Model file for the job. Use its own axes, mm. A direction names the side the tool comes from. Coordinates: 2 decimals unless noted, no trailing zeros. Order: outer loops, then holes, each group sorted by start corner. A loop starts at its lowest first (then second) coordinate and runs counter-clockwise, first axis right, second up. Notation, with made-up numbers: (4, 48.5) -> (10, 48.5) arc R25 ccw to (10, 83.5) -> close; hole circle Ø7 at (-17, 8.25). An arc over 180 degrees is marked (long way). Return JSON: item names as keys, results as strings. Group by question number.
1) Probe line 1 (Y direction, x = 31, z = 95); line 2 (Z direction, x = 273, y = 10.5) (3 decimals); line 3 (Y direction, x = 35.5, z = 82). List the from-to ranges inside material, lowest first.
2) Which spindle directions (+Z, -Z, +X, -X, +Y, -Y) get a long thin tool onto all of the face, cutting with end or side? Do faces 1 (the flat face through (302, -1, 0)), 2 (the flat face through (-10, 10, 0)), 3 (the flat face through (455, -10, 0)), 4 (the flat face through (454, 10, 127)). Say none if no direction does.
3) Flat gauge pins, fed straight in: pin 1 (1.5 mm diameter, centred on x = 292, z = 116, fed in from -Y); pin 2 (2 mm diameter, centred on y = -8.5, z = 73, fed in from +X); pin 3 (4 mm diameter, centred on x = -4, y = -5.5, fed in from +Z) (3 decimals); pin 4 (4 mm diameter, centred on x = 79.5, z = 90.5, fed in from +Y). Where does each tip first touch, or does it go through?
4) Cut at B-B (x = 120.5). Write the cut outline in (y, z) (3 decimals).
5) Pull direction X, two halves, no side cores. Call faces 5 (the flat face through (111, -1, 127)), 6 (the flat face through (219, 0, 130.175)): +X half, -X half, draft (parallel to the pull), parting line (faces both ways), or undercut.
6) Cut at A-A (z = 67). State how many separate pieces and enclosed holes the cut face has, and give its area (3 significant figures).
from build123d import *

# Parameters (mm, degrees)
SKETCH1_R           = 12.7
BOSS_EXTRUDE1_DEPTH = 127
LPATTERN1_COUNT     = 15
LPATTERN1_PITCH     = 31.75
SKETCH2_W           = 469.9
SKETCH2_H           = 25.4
BOSS_EXTRUDE2_DEPTH = 3.175
SKETCH3_R           = 8.255
CUT_EXTRUDE1_DEPTH  = 477.41930324


with BuildPart() as part:
    # Sketch1 → Boss-Extrude1 (new body)
    with BuildSketch(Plane.XY):
        Circle(SKETCH1_R)
    extrude(amount=BOSS_EXTRUDE1_DEPTH)


with BuildPart() as lpattern1_1:
    # LPattern1: pattern copy
    add(part.part.moved(Location(Vector(1, 0, 0) * (1 * LPATTERN1_PITCH))))


with BuildPart() as lpattern1_2:
    # LPattern1: pattern copy
    add(part.part.moved(Location(Vector(1, 0, 0) * (2 * LPATTERN1_PITCH))))


with BuildPart() as lpattern1_3:
    # LPattern1: pattern copy
    add(part.part.moved(Location(Vector(1, 0, 0) * (3 * LPATTERN1_PITCH))))


with BuildPart() as lpattern1_4:
    # LPattern1: pattern copy
    add(part.part.moved(Location(Vector(1, 0, 0) * (4 * LPATTERN1_PITCH))))


with BuildPart() as lpattern1_5:
    # LPattern1: pattern copy
    add(part.part.moved(Location(Vector(1, 0, 0) * (5 * LPATTERN1_PITCH))))


with BuildPart() as lpattern1_6:
    # LPattern1: pattern copy
    add(part.part.moved(Location(Vector(1, 0, 0) * (6 * LPATTERN1_PITCH))))


with BuildPart() as lpattern1_7:
    # LPattern1: pattern copy
    add(part.part.moved(Location(Vector(1, 0, 0) * (7 * LPATTERN1_PITCH))))


with BuildPart() as lpattern1_8:
    # LPattern1: pattern copy
    add(part.part.moved(Location(Vector(1, 0, 0) * (8 * LPATTERN1_PITCH))))


with BuildPart() as lpattern1_9:
    # LPattern1: pattern copy
    add(part.part.moved(Location(Vector(1, 0, 0) * (9 * LPATTERN1_PITCH))))


with BuildPart() as lpattern1_10:
    # LPattern1: pattern copy
    add(part.part.moved(Location(Vector(1, 0, 0) * (10 * LPATTERN1_PITCH))))


with BuildPart() as lpattern1_11:
    # LPattern1: pattern copy
    add(part.part.moved(Location(Vector(1, 0, 0) * (11 * LPATTERN1_PITCH))))


with BuildPart() as lpattern1_12:
    # LPattern1: pattern copy
    add(part.part.moved(Location(Vector(1, 0, 0) * (12 * LPATTERN1_PITCH))))


with BuildPart() as lpattern1_13:
    # LPattern1: pattern copy
    add(part.part.moved(Location(Vector(1, 0, 0) * (13 * LPATTERN1_PITCH))))


with BuildPart() as lpattern1_14:
    # LPattern1: pattern copy
    add(part.part.moved(Location(Vector(1, 0, 0) * (14 * LPATTERN1_PITCH))))


with BuildPart() as part_1:
    add(part.part)

    add(lpattern1_1.part)  # Boss-Extrude2 merges LPattern1_1

    add(lpattern1_2.part)  # Boss-Extrude2 merges LPattern1_2

    add(lpattern1_3.part)  # Boss-Extrude2 merges LPattern1_3

    add(lpattern1_4.part)  # Boss-Extrude2 merges LPattern1_4

    add(lpattern1_5.part)  # Boss-Extrude2 merges LPattern1_5

    add(lpattern1_6.part)  # Boss-Extrude2 merges LPattern1_6

    add(lpattern1_7.part)  # Boss-Extrude2 merges LPattern1_7

    add(lpattern1_8.part)  # Boss-Extrude2 merges LPattern1_8

    add(lpattern1_9.part)  # Boss-Extrude2 merges LPattern1_9

    add(lpattern1_10.part)  # Boss-Extrude2 merges LPattern1_10

    add(lpattern1_11.part)  # Boss-Extrude2 merges LPattern1_11

    add(lpattern1_12.part)  # Boss-Extrude2 merges LPattern1_12

    add(lpattern1_13.part)  # Boss-Extrude2 merges LPattern1_13

    add(lpattern1_14.part)  # Boss-Extrude2 merges LPattern1_14
    # Sketch2 → Boss-Extrude2 (add)
    with BuildSketch(Plane.XY.offset(127)):
        with Locations((222.25, 0)):
            Rectangle(SKETCH2_W, SKETCH2_H)
    boss_extrude2 = extrude(amount=BOSS_EXTRUDE2_DEPTH)

    # Mirror1: Boss-Extrude2 across plane
    add(boss_extrude2.mirror(Plane.XY.offset(63.5)))

    # Sketch3 → Cut-Extrude1 (cut, through all)
    with BuildSketch(Plane.XY.offset(130.175)):
        with Locations((31.75, 0)):
            Circle(SKETCH3_R)
        Polygon((7.332348419, 0), (3.666174209, 6.35), (-3.666174209, 6.35), (-7.332348419, 0), (-3.666174209, -6.35), (3.666174209, -6.35), align=None)
    extrude(amount=-CUT_EXTRUDE1_DEPTH, mode=Mode.SUBTRACT)


solid = part_1.part
Answers below:
{
 "1": {"line 1": "y = -12.68 to -8.22, 8.22 to 12.68", "line 2": "z = -3.175 to 0, 127 to 130.175", "line 3": "y = -12.13 to -7.35, 7.35 to 12.13"},
 "2": {"face 1": "none", "face 2": "-X, +Y", "face 3": "+X, -Y", "face 4": "+X, +Y"},
 "3": {"pin 1": "stops at y = -11.45", "pin 2": "stops at x = 454.75", "pin 3": "stops at z = 130.175", "pin 4": "passes through"},
 "4": {"outline": "(-12.7, -3.175) -> (12.7, -3.175) -> (12.7, 0) -> (10.911, 0) -> (10.911, 127) -> (12.7, 127) -> (12.7, 130.175) -> (-12.7, 130.175) -> (-12.7, 127) -> (-10.911, 127) -> (-10.911, 0) -> (-12.7, 0) -> close"},
 "5": {"face 5": "undercut", "face 6": "draft"},
 "6": {"separate pieces": "15", "enclosed holes": "2", "area": "7,250 mm^2"}
}
